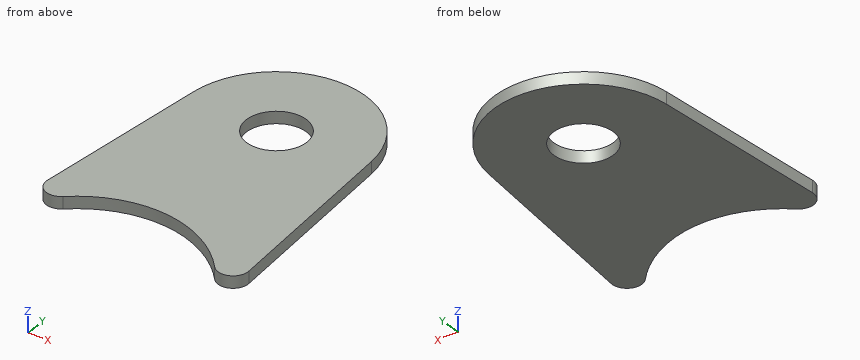
from build123d import *

# Parameters (mm, degrees)
SKETCH1_R           = 3.175
BOSS_EXTRUDE1_DEPTH = 0.635
SKETCH2_R           = 12.7
CUT_EXTRUDE4_DEPTH  = 212.524238452
CUT_EXTRUDE5_DEPTH  = 37.22284017
FILLET1_R           = 1.5875


with BuildPart() as part:
    # Sketch1 → Boss-Extrude1 (new, symmetric)
    with BuildSketch(Plane.XY):
        with BuildLine():
            Line((-9.484545184, 0.876942223), (-12.7, -33.89972345))
            Line((-12.7, -33.89972345), (12.7, -33.89972345))
            Line((12.7, -33.89972345), (9.484545184, 0.876942223))
            ThreePointArc((9.484545184, 0.876942223), (0, 9.525), (-9.484545184, 0.876942223))
        make_face()
        Circle(SKETCH1_R, mode=Mode.SUBTRACT)
    extrude(amount=BOSS_EXTRUDE1_DEPTH, both=True)

    # Sketch2 → Cut-Extrude4 (cut, through all)
    with BuildSketch(Plane(origin=(11.360273025, -110.358999973, -171.966950351), x_dir=(0.9980881037002614, 0.025903655155534222, 0.05611718009308436), z_dir=(-0.06180716474340577, 0.4198866087842844, 0.9054695523042258))):
        Circle(SKETCH2_R)
    extrude(amount=CUT_EXTRUDE4_DEPTH, mode=Mode.SUBTRACT)


with BuildPart() as cut_extrude4_kept_piece:
    # of the separate pieces the step leaves, the one the design keeps (cut_extrude4_pieces_kept)
    add(part.part.solids().sort_by_distance((-9.484545184, 0.876942223, 0.635))[0])

    # Sketch3 → Cut-Extrude5 (cut, through all)
    with BuildSketch(Plane.XY.offset(0.635)):
        with BuildLine():
            Line((-11.744890387, -23.569760946), (-12.986106665, -32.169096948))
            Line((-12.986106665, -32.169096948), (12.819749994, -35.194876316))
            Line((12.819749994, -35.194876316), (11.371919396, -19.535903157))
            ThreePointArc((11.371919396, -19.535903157), (10.419687683, -21.139836428), (8.599708374, -20.731152577))
            add(Edge.make_bspline(
                [(8.599708374, -20.731152577), (-3.74867157, -6.707106034), (-11.744890387, -23.569760946)],
                knots=[2.192806487, 2.192806487, 2.192806487, 4.076762859, 4.076762859, 4.076762859], degree=2, weights=[1, 0.588189372, 1]))
        make_face()
    extrude(amount=-CUT_EXTRUDE5_DEPTH, mode=Mode.SUBTRACT)

    # Fillet1
    fillet1_edges = [cut_extrude4_kept_piece.edges().sort_by_distance(p)[0] for p in [
        (-11.744890387, -23.569760946, 0),
    ]]
    fillet(fillet1_edges, radius=FILLET1_R)


solid = cut_extrude4_kept_piece.part
For this review, take the finished solid that the model builds, in its own axes (mm). Round coordinates to 2 decimals unless told otherwise and drop trailing zeros. Loops run counter-clockwise (first coordinate to the right, second up) from the corner with the lowest first, then second, coordinate; pieces in that order, holes last. Notation, with made-up numbers: (-20.75, 8) - (5.25, 8) arc R34 cw to (5.25, 45) - close; hole circle Ø7 at (45.5, 14.5). An arc over 180 degrees is marked (long way). One line per item, written item: value. Start each with the question number.
Item 1: For L1, parallel to Y at x = 0, z = 0.3 (3 decimals); L2, parallel to Y at x = -2.5, z = -0.45; L3, parallel to X at y = -18.5, z = 0.15, list the stretches that pass through material, from the lowest coordinate up.
Item 2: Take a section at B-B (y = -10.5). Give the boundary of the cut face in (x, z) (3 decimals).
Item 3: Take a section at C-C (y = 4). Give the boundary of the cut face in (x, z) (3 decimals), plus the area to 3 significant figures.
Item 4: Clearance check with a flat-ended pin moving along its axis: pin 1 Ø4 at (x, y) = (0, 0) entering from +Z (3 decimals). State where the tip first meets the part, or that it passes through.
Item 5: Take a section at A-A (y = -0.5). Give the boundary of the cut face in (x, z) (3 decimals), plus the area to 3 significant figures.
Answer below:
1. L1: y = -16.347 to -3.175, 3.175 to 9.525
1. L2: y = -16.45 to -1.96, 1.96 to 9.19
1. L3: x = -11.2 to -7.55, 6.09 to 11.28
2. outline: (-10.536, -0.635) - (10.536, -0.635) - (10.536, 0.635) - (-10.536, 0.635) - close
3. outline: (-8.644, -0.635) - (8.644, -0.635) - (8.644, 0.635) - (-8.644, 0.635) - close
3. area: 22.0 mm2
4. pin 1: passes through
5. outline: (-9.612, -0.635) - (-3.135, -0.635) - (-3.135, 0.635) - (-9.612, 0.635) - close; (3.135, -0.635) - (9.612, -0.635) - (9.612, 0.635) - (3.135, 0.635) - close
5. area: 16.5 mm2
